Design review of the part built by this model. Coordinates are the model's own, in mm. A direction names the side the tool comes from. Coordinates: 2 decimals unless noted, no trailing zeros. Loops run counter-clockwise (first coordinate to the right, second up) from the corner with the lowest first, then second, coordinate; pieces in that order, holes last. Notation, with made-up numbers: (-15.5, 81) -> (-9.5, 81) arc R6 ccw to (-9.5, 87) -> close; hole circle Ø5 at (8.5, -13.75). An arc over 180 degrees is marked (long way). Answer in a Markdown table with one row per item.
```python
from build123d import *

# Parameters (mm, degrees)
M5X0_8_TAPPED_HOLE1_D                               = 4.2
M5X0_8_TAPPED_HOLE1_DEPTH                           = 46.99
M5X0_8_TAPPED_HOLE1_TIP                             = 1.2618073
CIRPATTERN1_COUNT                                   = 3
CBORE_FOR_00_BINDING_HEAD_MACHINE_SCREW_D           = 1.397
CBORE_FOR_00_BINDING_HEAD_MACHINE_SCREW_DEPTH       = 6.35
CBORE_FOR_00_BINDING_HEAD_MACHINE_SCREW_CBORE_D     = 7.874
CBORE_FOR_00_BINDING_HEAD_MACHINE_SCREW_CBORE_DEPTH = 0.254
CBORE_FOR_00_BINDING_HEAD_MACHINE_SCREW_TIP         = 0.419701142
SKETCH2_R                                           = 61.6585
EXTRUDE1_DEPTH                                      = 1.016


with BuildPart() as part:
    # Sketch1 → Revolve1 (revolve)
    with BuildSketch(Plane.XY, mode=Mode.PRIVATE) as revolve1_sk:
        with BuildLine():
            Line((0, 0), (62.4967, 0))
            Line((62.4967, 0), (62.4967, 27.6606))
            Line((62.4967, 27.6606), (56.1467, 34.0106))
            Line((56.1467, 34.0106), (9.955892816, 34.0106))
            ThreePointArc((9.955892816, 34.0106), (7.551444809, 28.459428687), (2.3876, 25.307987753))
            Line((2.3876, 25.307987753), (2.3876, 24.6126))
            Line((2.3876, 24.6126), (0, 24.6126))
            Line((0, 24.6126), (0, 0))
        make_face()
    revolve(revolve1_sk.sketch.rotate(Axis((0, 23.9776, 0), (0, -1, 0)), 180), axis=Axis((0, 23.9776, 0), (0, -1, 0)))  # turned: the seam where the file's is

    # M5x0.8 Tapped Hole1
    with Locations(Plane(origin=(62.4967, 8.0772, 0), x_dir=(0, 0, 1), z_dir=(1, 0, 0))):
        with Locations((0, 0)):
            Hole(M5X0_8_TAPPED_HOLE1_D / 2, depth=M5X0_8_TAPPED_HOLE1_DEPTH)
            with Locations((0, 0, -(M5X0_8_TAPPED_HOLE1_DEPTH + M5X0_8_TAPPED_HOLE1_TIP / 2))):  # 118° drill point
                Cone(0, M5X0_8_TAPPED_HOLE1_D / 2, M5X0_8_TAPPED_HOLE1_TIP, mode=Mode.SUBTRACT)

    # Sketch5 → M3x0.5 Tapped Hole1 (revolve, cut)
    with BuildSketch(Plane(origin=(-15.875, 34.0106, 0), x_dir=(0, 0, 1), z_dir=(1, 0, 0))):
        Polygon((0, 0), (0, 10.403075774), (1.25, 9.652), (1.25, 0), align=None)
    m3x0_5_tapped_hole1 = revolve(axis=Axis((-15.875, 40.3606, 0), (0, -1, 0)), mode=Mode.SUBTRACT)

    # CirPattern1: M3x0.5 Tapped Hole1 ×3 about axis
    cirpattern1_axis = Axis((0, 0, 0), (0, 1, 0))
    for i in range(1, CIRPATTERN1_COUNT):
        add(m3x0_5_tapped_hole1.rotate(cirpattern1_axis, i * 360 / CIRPATTERN1_COUNT), mode=Mode.SUBTRACT)

    # CBORE for #00 Binding Head Machine Screw1
    with Locations(Plane(origin=(62.4967, 8.0772, 0), x_dir=(0, 0, 1), z_dir=(1, 0, 0))):
        with Locations((0, 0)):
            CounterBoreHole(CBORE_FOR_00_BINDING_HEAD_MACHINE_SCREW_D / 2, CBORE_FOR_00_BINDING_HEAD_MACHINE_SCREW_CBORE_D / 2, CBORE_FOR_00_BINDING_HEAD_MACHINE_SCREW_CBORE_DEPTH, depth=CBORE_FOR_00_BINDING_HEAD_MACHINE_SCREW_DEPTH)
            with Locations((0, 0, -(CBORE_FOR_00_BINDING_HEAD_MACHINE_SCREW_DEPTH + CBORE_FOR_00_BINDING_HEAD_MACHINE_SCREW_TIP / 2))):  # 118° drill point
                Cone(0, CBORE_FOR_00_BINDING_HEAD_MACHINE_SCREW_D / 2, CBORE_FOR_00_BINDING_HEAD_MACHINE_SCREW_TIP, mode=Mode.SUBTRACT)

    # Sketch2 → Extrude1 (add)
    with BuildSketch(Plane.XZ):
        with Locations(Location((0, 0, 0), (0, 0, 180))):  # turned: the seam where the file's is
            Circle(SKETCH2_R)
    extrude(amount=EXTRUDE1_DEPTH)


solid = part.part
```
(1) To check wall thickness, follow probe 1 along Z at (x, y) = (0, 25.1); probe 2 along Y at (x, z) = (62, 0); probe 3 along X at (y, z) = (32, 8.5). State the ranges of each line that lie inside material, in increasing order.
Evaluation:
| item | result |
|---|---|
| probe 1 | z = -62.5 to -2.39, 2.39 to 62.5 |
| probe 2 | y = 0 to 5.98, 10.18 to 28.16 |
| probe 3 | x = -57.53 to -4.33, 4.33 to 57.53 |
(2) For pin 1 (5 mm diameter, centred on y = 8.08, z = 0, fed in from +X); pin 2 (1.5 mm diameter, centred on y = 30, z = 17, fed in from -X); pin 3 (8 mm diameter, centred on x = 46.5, y = 12, fed in from -Z), all flat-tipped, find the tip position at first contact; note any pin that passes through.
Evaluation:
| item | result |
|---|---|
| pin 1 | stops at x = 62.24 |
| pin 2 | stops at x = -58.52 |
| pin 3 | stops at z = -45.82 |
(3) Take a section at B-B on y = 16. Give the boundary of the cut face in (x, z).
Evaluation:
| item | result |
|---|---|
| outline | circle Ø124.99 at (0, 0) |
(4) Tool access review of faces 4 (the cylindrical face through (0.52, 24.96, 2.33)), 5 (the cylindrical face through (8.027, -0.501, -61.134)), 6 (the cylindrical face through (38.5, 6, 0.3)): name each direction out of +Z, -Z, +X, -X, +Y, -Y from which nothing blocks a thin tool from reaching the whole face with its end or side.
Evaluation:
| item | result |
|---|---|
| face 4 | +Y |
| face 5 | -Y |
| face 6 | +X |
(5) Take a section at A-A on x = 0. Give the boundary of the cut face in (y, z), and give its area (3 significant figures).
Evaluation:
| item | result |
|---|---|
| outline | (-1.02, -61.66) -> (0, -61.66) -> (0, -62.5) -> (27.66, -62.5) -> (34.01, -56.15) -> (34.01, -9.96) arc R10.01 cw to (25.31, -2.39) -> (24.61, -2.39) -> (24.61, 2.39) -> (25.31, 2.39) arc R10.01 cw to (34.01, 9.96) -> (34.01, 56.15) -> (27.66, 62.5) -> (0, 62.5) -> (0, 61.66) -> (-1.02, 61.66) -> close |
| area | 4,200 mm² |
(6) Draft analysis for pull direction X (two halves, no side actions). For faces 1 (the flat face through (1, -1.016, -1)), 2 (the flat face through (62.243, 10, 2)), 3 (the flat face through (0, 24.613, 0)), state which applies: pulls with the +X half, pulls with the -X half, needs draft (parallel to the pull), parting line crosses it, or undercut.
Evaluation:
| item | result |
|---|---|
| face 1 | needs draft |
| face 2 | pulls with the +X half |
| face 3 | undercut |
